```python
from build123d import *

# Parameters (mm, degrees)
F0_R     = 4.75
F1_DEPTH = 2
F2_DEPTH = 4


# Not quite as in the source:
# - a fillet or chamfer that OpenCascade refuses, or shapes differently, is made with other operations: its cross-section is extruded or revolved along the edge and cut away or added
# - a feature names something its author has since deleted; it is built from what else it names


with BuildPart() as f1:
    # F0 (on Top) → F1 (new body)
    with BuildSketch(Plane.XY):
        Circle(F0_R)
        with BuildLine():
            ThreePointArc((-0.5, -3.9686269666), (-2.8284271247, -2.8284271247), (-3.9686269666, -0.5))
            Line((-3.9686269666, -0.5), (-2.7549954628, -0.5))
            Line((-2.7549954628, -0.5), (-0.5, -0.5))
            Line((-0.5, -0.5), (-0.5, -2.7549954628))
            Line((-0.5, -2.7549954628), (-0.5, -3.9686269666))
        make_face(mode=Mode.SUBTRACT)
        with BuildLine():
            Line((0.5, -0.5), (2.7549954628, -0.5))
            Line((2.7549954628, -0.5), (3.9686269666, -0.5))
            ThreePointArc((3.9686269666, -0.5), (2.8284271247, -2.8284271247), (0.5, -3.9686269666))
            Line((0.5, -3.9686269666), (0.5, -2.7549954628))
            Line((0.5, -2.7549954628), (0.5, -0.5))
        make_face(mode=Mode.SUBTRACT)
        with BuildLine():
            Line((-2.7549954628, 0.5), (-3.9686269666, 0.5))
            ThreePointArc((-3.9686269666, 0.5), (-2.8284271247, 2.8284271247), (-0.5, 3.9686269666))
            Line((-0.5, 3.9686269666), (-0.5, 2.7549954628))
            Line((-0.5, 2.7549954628), (-0.5, 0.5))
            Line((-0.5, 0.5), (-2.7549954628, 0.5))
        make_face(mode=Mode.SUBTRACT)
        with BuildLine():
            Line((3.9686269666, 0.5), (2.7549954628, 0.5))
            Line((2.7549954628, 0.5), (0.5, 0.5))
            Line((0.5, 0.5), (0.5, 2.7549954628))
            Line((0.5, 2.7549954628), (0.5, 3.9686269666))
            ThreePointArc((0.5, 3.9686269666), (2.8284271247, 2.8284271247), (3.9686269666, 0.5))
        make_face(mode=Mode.SUBTRACT)
        with BuildLine():
            Line((-2.7549954628, -0.5), (-3.9686269666, -0.5))
            ThreePointArc((-3.9686269666, -0.5), (-2.8284271247, -2.8284271247), (-0.5, -3.9686269666))
            Line((-0.5, -3.9686269666), (-0.5, -2.7549954628))
            Line((-0.5, -2.7549954628), (-0.5, -0.5))
            Line((-0.5, -0.5), (-2.7549954628, -0.5))
        make_face()
        with BuildLine():
            ThreePointArc((-0.5, 3.9686269666), (-2.8284271247, 2.8284271247), (-3.9686269666, 0.5))
            Line((-3.9686269666, 0.5), (-2.7549954628, 0.5))
            Line((-2.7549954628, 0.5), (-0.5, 0.5))
            Line((-0.5, 0.5), (-0.5, 2.7549954628))
            Line((-0.5, 2.7549954628), (-0.5, 3.9686269666))
        make_face()
        with BuildLine():
            Line((0.5, 0.5), (2.7549954628, 0.5))
            Line((2.7549954628, 0.5), (3.9686269666, 0.5))
            ThreePointArc((3.9686269666, 0.5), (2.8284271247, 2.8284271247), (0.5, 3.9686269666))
            Line((0.5, 3.9686269666), (0.5, 2.7549954628))
            Line((0.5, 2.7549954628), (0.5, 0.5))
        make_face()
        with BuildLine():
            Line((3.9686269666, -0.5), (2.7549954628, -0.5))
            Line((2.7549954628, -0.5), (0.5, -0.5))
            Line((0.5, -0.5), (0.5, -2.7549954628))
            Line((0.5, -2.7549954628), (0.5, -3.9686269666))
            ThreePointArc((0.5, -3.9686269666), (2.8284271247, -2.8284271247), (3.9686269666, -0.5))
        make_face()
    extrude(amount=F1_DEPTH)

    # F0 (on Top) → F2 (join)
    with BuildSketch(Plane.XY):
        with BuildLine():
            ThreePointArc((-0.5, 3.9686269666), (-2.8284271247, 2.8284271247), (-3.9686269666, 0.5))
            Line((-3.9686269666, 0.5), (-2.7549954628, 0.5))
            Line((-2.7549954628, 0.5), (-0.5, 0.5))
            Line((-0.5, 0.5), (-0.5, 2.7549954628))
            Line((-0.5, 2.7549954628), (-0.5, 3.9686269666))
        make_face()
        with BuildLine():
            Line((-2.7549954628, -0.5), (-3.9686269666, -0.5))
            ThreePointArc((-3.9686269666, -0.5), (-2.8284271247, -2.8284271247), (-0.5, -3.9686269666))
            Line((-0.5, -3.9686269666), (-0.5, -2.7549954628))
            Line((-0.5, -2.7549954628), (-0.5, -0.5))
            Line((-0.5, -0.5), (-2.7549954628, -0.5))
        make_face()
        with BuildLine():
            Line((3.9686269666, -0.5), (2.7549954628, -0.5))
            Line((2.7549954628, -0.5), (0.5, -0.5))
            Line((0.5, -0.5), (0.5, -2.7549954628))
            Line((0.5, -2.7549954628), (0.5, -3.9686269666))
            ThreePointArc((0.5, -3.9686269666), (2.8284271247, -2.8284271247), (3.9686269666, -0.5))
        make_face()
        with BuildLine():
            Line((0.5, 0.5), (2.7549954628, 0.5))
            Line((2.7549954628, 0.5), (3.9686269666, 0.5))
            ThreePointArc((3.9686269666, 0.5), (2.8284271247, 2.8284271247), (0.5, 3.9686269666))
            Line((0.5, 3.9686269666), (0.5, 2.7549954628))
            Line((0.5, 2.7549954628), (0.5, 0.5))
        make_face()
    extrude(amount=-F2_DEPTH)

    # F3: fillet of radius 4.7 on 1 edges, made by hand

    # F3_s1 → F3_t2 (revolve, cut)
    with BuildSketch(Plane.XZ):
        with BuildLine():
            ThreePointArc((4.75, 0), (3.0708715265, 1.4701318924), (0.9029231877, 2))
            Line((0.9029231877, 2), (4.75, 2))
            Line((4.75, 2), (4.75, 0))
        make_face()
    revolve(axis=Axis((0, 0, 2), (0, 0, 1)), mode=Mode.SUBTRACT)


solid = f1.part
```
The model under review builds one solid part; all positions refer to its coordinate system, in mm. A direction names the side the tool comes from. Coordinates: 2 decimals unless noted, no trailing zeros. Write each loop counter-clockwise with the first axis right and the second up, starting at its lowest first coordinate (ties: lowest second). Pieces come first, ordered by that corner, then holes. Notation, with made-up numbers: (3.25, 38.5) - (12.25, 38.5) arc R18 ccw to (12.25, 57.5) - close; hole circle Ø8 at (26, 67). An arc over 180 degrees is marked (long way). Answer in a Markdown table with one row per item. Add a question column.
Q1. Draft analysis for pull direction Y (two halves, no side actions). For faces 5 (the face through (0, 0, 0)), 6 (the face through (2, 2, -4)), 7 (the face through (-2.802, 2.854, -1.972)), state which applies: +Y half, -Y half, draft (parallel to the pull), parting line (faces both ways), or undercut.
Q2. Consider section A-A on z = -1. Give the boundary of the cut face in (x, y), then the cut area to 3 significant figures.
Q3. To check wall thickness, follow line 1 along Z through (x, y) = (0, 0); line 2 along X through (y, z) = (-2.5, -2.25). State the ranges of each line that lie inside material, in increasing order. Write a range as from..to.
Q4. For faces 1 (the face through (2, -0.5, -2)), 2 (the face through (0.5, -2, -2)), 3 (the face through (2.854, 2.802, -1.972)), 4 (the face through (2.802, -2.854, -1.972)), list the 3-axis set-ups (+Z, -Z, +X, -X, +Y, -Y) from which the entire face can be reached by the end or side of a thin tool; tool diameter is ignored.
Q5. Clearance check with flat-ended pins moving along their axes: pin 1 (3 mm diameter, centred on x = 1.5, z = -1, fed in from +Y); pin 2 (1.7 mm diameter, centred on y = 2, z = -1.5, fed in from +X); pin 3 (3 mm diameter, centred on y = 1.5, z = -2.5, fed in from -X). State where each tip first meets the part, or that it passes through.
Answers below:
| question | item | result |
|---|---|---|
| 1 | face 5 | undercut |
| 1 | face 6 | draft |
| 1 | face 7 | +Y half |
| 2 | outline | (-3.97, -0.5) arc R4 ccw to (-0.5, -3.97) - (-0.5, -0.5) - close; (-3.97, 0.5) - (-0.5, 0.5) - (-0.5, 3.97) arc R4 ccw to start; (0.5, -3.97) arc R4 ccw to (3.97, -0.5) - (0.5, -0.5) - close; (0.5, 0.5) - (3.97, 0.5) arc R4 ccw to (0.5, 3.97) - close |
| 2 | area | 35.3 mm² |
| 3 | line 1 | 0..2 |
| 3 | line 2 | -3.12..-0.5, 0.5..3.12 |
| 4 | face 1 | -Z, +X, -X |
| 4 | face 2 | -Z, +Y, -Y |
| 4 | face 3 | -Z, +X, +Y |
| 4 | face 4 | -Z, +X, -Y |
| 5 | pin 1 | y = 4.73 |
| 5 | pin 2 | x = 3.83 |
| 5 | pin 3 | x = -3.97 |
